The model under review builds one solid part; all positions refer to its coordinate system, in mm. Face numbers are marked on the shaded views. A direction names the side the tool comes from. Round coordinates to 2 decimals unless told otherwise and drop trailing zeros. Order: outer loops, then holes, each group sorted by start corner. A loop starts at its lowest first (then second) coordinate and runs counter-clockwise, first axis right, second up. Notation, with made-up numbers: (1.5, -19) - (5.5, -19) arc R20 cw to (5.5, 10) - close; hole circle Ø8 at (30, 82.5). An arc over 180 degrees is marked (long way). One line per question, with ' | ' between items. Start each with the question number.
Item 1: Tool access review of the marked faces 1 and 2: name each direction out of +Z, -Z, +X, -X, +Y, -Y from which nothing blocks a thin tool from reaching the whole face with its end or side.
Item 2: Add section B-B on x = 25. State the section outline as (y, z) points.
Item 3: Add section D-D on y = 2.25. State the section outline as (x, z) points.
Item 4: Insertion check: pin 1 Ø5.5 at (x, y) = (-25, 0) entering from +Z; pin 2 Ø2.5 at (y, z) = (0.5, 8.5) entering from -X; pin 3 Ø4 at (x, y) = (-7.5, 4) entering from +Z. Each pin has a flat end and moves straight along its axis. Give the tip position at first contact, or say it passes through.
Item 5: Add section A-A on z = 2.25. State the section outline as (x, y) points, and give its area (3 significant figures).
Item 6: Add section C-C on y = -0.5. State the section outline as (x, z) points.
Item 7: For L1, parallel to Y at x = 16.65, z = 3.3; L2, parallel to Y at x = 25, z = 1.6; L3, parallel to X at y = 0.75, z = 4.5, list the stretches that pass through material, from the lowest coordinate up. Write a range as [from, to].
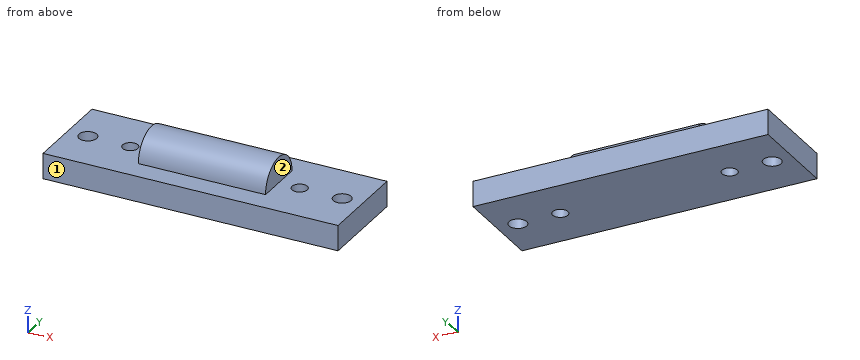
from build123d import *

# Parameters (mm, degrees)
F0_W     = 38
F0_H     = 18.5
F0_R     = 1.5
F0_W_2   = 10
F0_R_2   = 1.75
F1_DEPTH = 5
F2_W     = 25
F2_H     = 18.5
F3_DEPTH = 9.25
F5_DEPTH = 25


with BuildPart() as f1:
    # F0 (on Top) → F1 (new body)
    with BuildSketch(Plane.XY):
        Rectangle(F0_W, F0_H)
        with Locations((-16.65, 0)):
            Circle(F0_R, mode=Mode.SUBTRACT)
        with Locations((16.65, 0)):
            Circle(F0_R, mode=Mode.SUBTRACT)
        with Locations((24, 0)):
            Rectangle(F0_W_2, F0_H)
        with Locations((25, 0)):
            Circle(F0_R_2, mode=Mode.SUBTRACT)
        with Locations((-24, 0)):
            Rectangle(F0_W_2, F0_H)
        with Locations((-25, 0)):
            Circle(F0_R_2, mode=Mode.SUBTRACT)
    extrude(amount=F1_DEPTH)

    # F2 (on face) → F3 (join)
    with BuildSketch(Plane.XY.offset(5)):
        Rectangle(F2_W, F2_H)
    extrude(amount=F3_DEPTH)

    # F4 (on face) → F5 (cut)
    with BuildSketch(Plane.YZ.offset(12.5)):
        with BuildLine():
            ThreePointArc((-4.923553, 5), (0.07586, 10.076588), (5.075274, 5))
            Line((5.075274, 5), (9.25, 5))
            Line((9.25, 5), (9.25, 14.25))
            Line((9.25, 14.25), (-9.25, 14.25))
            Line((-9.25, 14.25), (-9.25, 5))
            Line((-9.25, 5), (-4.923553, 5))
        make_face()
    extrude(amount=-F5_DEPTH, mode=Mode.SUBTRACT)


solid = f1.part
Determined:
1) face 1: +Z, -Z, +X, -X, -Y | face 2: +Z, +X, +Y, -Y
2) outline: (-9.25, 0) - (-1.75, 0) - (-1.75, 5) - (-9.25, 5) - close; (1.75, 0) - (9.25, 0) - (9.25, 5) - (1.75, 5) - close
3) outline: (-29, 0) - (29, 0) - (29, 5) - (12.5, 5) - (12.5, 9.58) - (-12.5, 9.58) - (-12.5, 5) - (-29, 5) - close
4) pin 1: z = 5 | pin 2: x = -12.5 | pin 3: z = 9.69
5) outline: (-29, -9.25) - (29, -9.25) - (29, 9.25) - (-29, 9.25) - close; hole circle Ø3.5 at (-25, 0); hole circle Ø3 at (-16.65, 0); hole circle Ø3 at (16.65, 0); hole circle Ø3.5 at (25, 0) | area: 1,040 mm2
6) outline: (-29, 0) - (-26.68, 0) - (-26.68, 5) - (-29, 5) - close; (-23.32, 0) - (-18.06, 0) - (-18.06, 5) - (-23.32, 5) - close; (-15.24, 0) - (15.24, 0) - (15.24, 5) - (12.5, 5) - (12.5, 10.04) - (-12.5, 10.04) - (-12.5, 5) - (-15.24, 5) - close; (18.06, 0) - (23.32, 0) - (23.32, 5) - (18.06, 5) - close; (26.68, 0) - (29, 0) - (29, 5) - (26.68, 5) - close
7) L1: [-9.25, -1.5], [1.5, 9.25] | L2: [-9.25, -1.75], [1.75, 9.25] | L3: [-29, -26.58], [-23.42, -17.95], [-15.35, 15.35], [17.95, 23.42], [26.58, 29]
